Check sheet for the modelled part. Datum: model origin and axes. Units: mm. A direction names the side the tool comes from. Round coordinates to 2 decimals unless told otherwise and drop trailing zeros. Order: outer loops, then holes, each group sorted by start corner. A loop starts at its lowest first (then second) coordinate and runs counter-clockwise, first axis right, second up.
```python
from build123d import *

# Parameters (mm, degrees)
F1_DEPTH = 360
F3_DEPTH = 25.4
F4_DEPTH = 120


with BuildPart() as f1:
    # F0 (on Front) → F1 (new body)
    with BuildSketch(Plane.XZ):
        Polygon((260.316399, -285), (260.316399, 285), (-339.683601, 285), (-339.683601, -285), (-139.683601, -285), (-139.683601, -160), (60.316399, -160), (60.316399, -285), align=None)
    extrude(amount=F1_DEPTH)

    # F2 (on face) → F3 (join)
    with BuildSketch(Plane.XY.offset(285)):
        Polygon((-159.683601, 0), (-339.683601, 0), (-339.683601, -180), align=None)
        Polygon((260.316399, 0), (80.316399, 0), (260.316399, -180), align=None)
    extrude(amount=F3_DEPTH)

    # F3_face (on face) → F4 (join)
    with BuildSketch(Plane(origin=(-279.683601, -60, 310.4), x_dir=(1, 0, 0), z_dir=(0, 0, 1))):
        Polygon((-60, -120), (120, 60), (-60, 60), align=None)
        Polygon((540, 60), (360, 60), (540, -120), align=None)
    extrude(amount=F4_DEPTH)


solid = f1.part
```
Item 1: Access from +Z, -Z, +X, -X, +Y, -Y to the whole of each face (thin tool, end or side, straight path). Record for faces 1 (the flat face through (-35, -217, 285)), 2 (the flat face through (260.316, -177, 68)), 3 (the flat face through (-41, -177, -160)).
Answer:
face 1: +Z, -Y
face 2: +Z, -Z, +X, +Y, -Y
face 3: -Z, +Y, -Y
Item 2: Scan lines: line 1 along X through (y, z) = (-83, -246.5); line 2 along Z through (x, y) = (19, -143); line 3 along Z through (x, y) = (-233.5, -118). Record each from-to range of solid material in increasing order.
Answer:
line 1: x = -339.68 to -139.68, 60.32 to 260.32
line 2: z = -160 to 285
line 3: z = -285 to 285
Item 3: Sectioned sample at D-D (y = -113). Record the cut outline in (x, z).
Answer:
outline: (-339.68, -285) - (-139.68, -285) - (-139.68, -160) - (60.32, -160) - (60.32, -285) - (260.32, -285) - (260.32, 430.4) - (193.32, 430.4) - (193.32, 285) - (-272.68, 285) - (-272.68, 430.4) - (-339.68, 430.4) - close
Item 4: Go/stop test with a flat-tipped pin: P1, Ø4, axis at x = 140.5, y = -250.5, coming from the +Z side. Record where the tip stops, or that it passes through.
Answer:
P1: stops at z = 285
Item 5: Sectioned sample at C-C (x = -94). Record the cut outline in (y, z), and give its area (3 significant figures).
Answer:
outline: (-360, -160) - (0, -160) - (0, 285) - (-360, 285) - close
area: 160,000 mm2
Item 6: Sectioned sample at B-B (y = -196.5). Record the cut outline in (x, z).
Answer:
outline: (-339.68, -285) - (-139.68, -285) - (-139.68, -160) - (60.32, -160) - (60.32, -285) - (260.32, -285) - (260.32, 285) - (-339.68, 285) - close
Item 7: Sectioned sample at A-A (z = 308.5). Record the cut outline in (x, y).
Answer:
outline: (-339.68, -180) - (-159.68, 0) - (-339.68, 0) - close; (80.32, 0) - (260.32, -180) - (260.32, 0) - close
Item 8: Release check for a two-part mould opening along X. For faces 4 (the flat face through (-339.684, -177, 68)), 5 (the flat face through (-35, 0, 68)), 6 (the flat face through (-139.684, -177, -223)) record: released by +X, released by -X, zero draft, split by the parting line, or undercut.
Answer:
face 4: released by -X
face 5: zero draft
face 6: undercut
